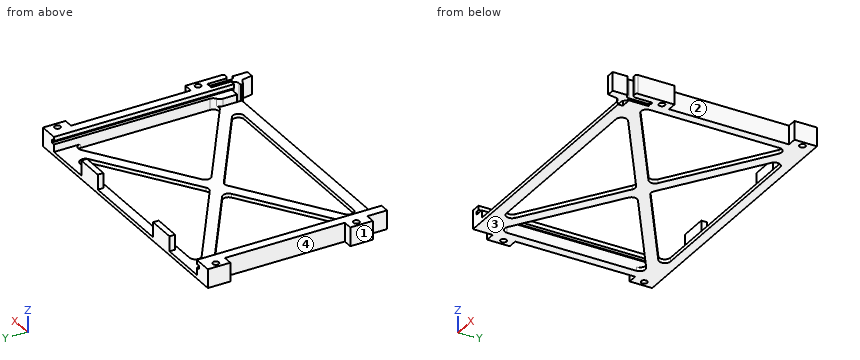
from build123d import *

# Parameters (mm, degrees)
BOSS_EXTRUDE1_DEPTH     = 10
SKETCH3_W               = 134.5
SKETCH3_H               = 1.8
CUT_EXTRUDE1_DEPTH      = 170.435828561
SKETCH5_W               = 140.5
SKETCH5_H               = 6
BOSS_EXTRUDE3_DEPTH     = 2
CUT_EXTRUDE2_DEPTH      = 170.435828561
FILLET1_R               = 3
BOSS_EXTRUDE2_OUTLINE_W = 5
BOSS_EXTRUDE2_OUTLINE_H = 12
BOSS_EXTRUDE2_OUTLINE_R = 1.6
BOSS_EXTRUDE2_DEPTH     = 10
SKETCH7_W               = 130.5
SKETCH7_H               = 5
CUT_EXTRUDE3_DEPTH      = 8
SKETCH8_W               = 15
SKETCH8_H               = 3
BOSS_EXTRUDE4_DEPTH     = 8
BOSS_EXTRUDE5_DEPTH     = 4
FILLET2_R               = 3


# Read off the part's stored shape, not the designer's step: Boss-Extrude2
with BuildPart() as part:
    # Sketch2 → Boss-Extrude1 (new body)
    with BuildSketch(Plane.XY):
        Polygon((2, 0), (-3, 0), (-3, 98.5), (137.5, 98.5), (137.5, 0), (132.5, 0), (132.5, 93.5), (2, 93.5), align=None)
    extrude(amount=BOSS_EXTRUDE1_DEPTH)

    # Sketch3 → Cut-Extrude1 (cut, through all)
    with BuildSketch(Plane.XZ):
        with Locations((67.25, 6.9)):
            Rectangle(SKETCH3_W, SKETCH3_H)
    extrude(amount=-CUT_EXTRUDE1_DEPTH, mode=Mode.SUBTRACT)

    # Sketch5 → Boss-Extrude3 (add)
    with BuildSketch(Plane(origin=(0, 0, 0), x_dir=(-1, 0, 0), z_dir=(0, 0, -1))):
        with Locations((-67.25, 3)):
            Rectangle(SKETCH5_W, SKETCH5_H)
        Polygon((-0.329295866, 8.49173588), (-130.829295866, 95.99173588), (-134.170704134, 91.00826412), (-3.670704134, 3.50826412), align=None)
        Polygon((-3.670704134, 95.99173588), (-134.170704134, 8.49173588), (-130.829295866, 3.50826412), (-0.329295866, 91.00826412), align=None)
    extrude(amount=-BOSS_EXTRUDE3_DEPTH)

    # Sketch4 → Cut-Extrude2 (cut, through all)
    with BuildSketch(Plane.XY):
        with BuildLine():
            ThreePointArc((132, 0), (133.457737974, 0.468990399), (134.368543856, 1.7))
            Line((134.368543856, 1.7), (135, 1.7))
            ThreePointArc((135, 1.7), (135.707106781, 1.992893219), (136, 2.7))
            Line((136, 2.7), (136, 13))
            Line((136, 13), (135.2, 13))
            Line((135.2, 13), (135.2, 2.5))
            Line((135.2, 2.5), (129.5, 2.5))
            Line((129.5, 2.5), (129.5, 0))
            Line((129.5, 0), (130.5, 0))
            Line((130.5, 0), (132, 0))
        make_face()
        with BuildLine():
            ThreePointArc((141.5, 2), (142.207106781, 2.292893219), (142.5, 3))
            Line((142.5, 3), (142.5, -0.5))
            Line((142.5, -0.5), (139.0272352, -0.5))
            Line((139.0272352, -0.5), (138.8, -0.5))
            ThreePointArc((138.8, -0.5), (137.385786438, 0.085786438), (136.8, 1.5))
            Line((136.8, 1.5), (136.8, 12))
            ThreePointArc((136.8, 12), (137.092893219, 12.707106781), (137.8, 13))
            Line((137.8, 13), (138.3, 13))
            ThreePointArc((138.3, 13), (138.653553391, 12.853553391), (138.8, 12.5))
            Line((138.8, 12.5), (138.8, 4))
            ThreePointArc((138.8, 4), (139.385786438, 2.585786438), (140.8, 2))
            Line((140.8, 2), (141.5, 2))
        make_face()
    extrude(amount=CUT_EXTRUDE2_DEPTH, mode=Mode.SUBTRACT)

    # Fillet1
    fillet1_edges = [part.edges().sort_by_distance(p)[0] for p in [
        (132.5, 89.888060199, 1),
        (72.636950218, 49.75, 1),
        (61.863049782, 49.75, 1),
        (67.25, 53.361939801, 1),
        (2, 89.888060199, 1),
        (127.113049782, 93.5, 1),
        (7.386950218, 6, 1),
        (2, 9.611939801, 1),
        (132.5, 9.611939801, 1),
        (67.25, 46.138060199, 1),
        (127.113049782, 6, 1),
        (7.386950218, 93.5, 1),
    ]]
    fillet(fillet1_edges, radius=FILLET1_R)

    # Boss-Extrude2 outline → Boss-Extrude2 (add)
    # profile 1 of 5: a face of its own
    with BuildSketch(Plane.XY):
        with BuildLine():
            Line((134.5, 1.7), (134.368543856, 1.7))
            ThreePointArc((134.368543856, 1.7), (133.457737974, 0.468990399), (132, 0))
            Line((132, 0), (130.5, 0))
            Line((130.5, 0), (130.5, -1.2))
            Line((130.5, -1.2), (134.0272352, -2.83697044))
            Line((134.0272352, -2.83697044), (135.0272352, -8.5))
            Line((135.0272352, -8.5), (139.0272352, -8.5))
            Line((139.0272352, -8.5), (139.0272352, -0.5))
            Line((139.0272352, -0.5), (138.8, -0.5))
            ThreePointArc((138.8, -0.5), (138.092893219, -0.370828693), (137.477124345, 1e-09))
            Line((137.477124345, 1e-09), (134.5, 0))
            Line((134.5, 0), (134.5, 1.7))
        make_face()
    # profile 2 of 5: a face of its own
    with BuildSketch(Plane.XY):
        with Locations((-5.5, 16.5)):
            Rectangle(BOSS_EXTRUDE2_OUTLINE_W, BOSS_EXTRUDE2_OUTLINE_H)
        with Locations((-5, 17.5)):
            Circle(BOSS_EXTRUDE2_OUTLINE_R, mode=Mode.SUBTRACT)
    # profile 3 of 5: a face of its own
    with BuildSketch(Plane.XY):
        with Locations((-5.5, 92.5)):
            Rectangle(BOSS_EXTRUDE2_OUTLINE_W, BOSS_EXTRUDE2_OUTLINE_H)
        with Locations((-5, 92.5)):
            Circle(BOSS_EXTRUDE2_OUTLINE_R, mode=Mode.SUBTRACT)
    # profile 4 of 5: a face of its own
    with BuildSketch(Plane.XY):
        with Locations((140, 92.5)):
            Rectangle(BOSS_EXTRUDE2_OUTLINE_W, BOSS_EXTRUDE2_OUTLINE_H)
        with Locations((139.5, 92.5)):
            Circle(BOSS_EXTRUDE2_OUTLINE_R, mode=Mode.SUBTRACT)
    # profile 5 of 5: a face of its own
    with BuildSketch(Plane.XY):
        with BuildLine():
            Line((137.8, 13), (138.3, 13))
            ThreePointArc((138.3, 13), (138.653553391, 12.853553391), (138.8, 12.5))
            Line((138.8, 12.5), (138.8, 4))
            ThreePointArc((138.8, 4), (139.385786438, 2.585786438), (140.8, 2))
            Line((140.8, 2), (141.5, 2))
            ThreePointArc((141.5, 2), (142.207106781, 2.292893219), (142.5, 3))
            Line((142.5, 3), (142.5, 22.5))
            Line((142.5, 22.5), (137.5, 22.5))
            Line((137.5, 22.5), (137.5, 12.953939201))
            ThreePointArc((137.5, 12.953939201), (137.648242301, 12.988417726), (137.8, 13))
        make_face()
        with Locations((139.5, 17.5)):
            Circle(BOSS_EXTRUDE2_OUTLINE_R, mode=Mode.SUBTRACT)
    extrude(amount=BOSS_EXTRUDE2_DEPTH)

    # Sketch7 → Cut-Extrude3 (cut)
    with BuildSketch(Plane.XY.offset(10)):
        with Locations((67.25, 96)):
            Rectangle(SKETCH7_W, SKETCH7_H)
    extrude(amount=-CUT_EXTRUDE3_DEPTH, mode=Mode.SUBTRACT)

    # Sketch8 → Boss-Extrude4 (add)
    with BuildSketch(Plane.XY.offset(2)):
        with Locations((34.5, 97)):
            Rectangle(SKETCH8_W, SKETCH8_H)
        with Locations((100, 97)):
            Rectangle(SKETCH8_W, SKETCH8_H)
    extrude(amount=BOSS_EXTRUDE4_DEPTH)

    # Sketch9 → Boss-Extrude5 (add)
    with BuildSketch(Plane.XY.offset(2)):
        with BuildLine():
            ThreePointArc((132.5, 15.235373856), (131.621320344, 13.114053512), (129.5, 12.235373856))
            Line((129.5, 12.235373856), (129.5, 2.5))
            Line((129.5, 2.5), (132.5, 2.5))
            Line((132.5, 2.5), (132.5, 15.235373856))
        make_face()
        with BuildLine():
            Line((2, 0), (5, 0))
            Line((5, 0), (5, 12.235373856))
            ThreePointArc((5, 12.235373856), (2.878679656, 13.114053512), (2, 15.235373856))
            Line((2, 15.235373856), (2, 0))
        make_face()
    extrude(amount=BOSS_EXTRUDE5_DEPTH)

    # Fillet2
    fillet2_edges = [part.edges().sort_by_distance(p)[0] for p in [
        (5, 12.235373856, 4),
        (129.5, 12.235373856, 4),
    ]]
    fillet(fillet2_edges, radius=FILLET2_R)


solid = part.part
Verification items for the finished model (mm, model axes). Face numbers are marked on the shaded views. A direction names the side the tool comes from. Give positions to 0.01 mm unless a question says otherwise; leave off trailing zeros. Loops run counter-clockwise (first coordinate to the right, second up) from the corner with the lowest first, then second, coordinate; pieces in that order, holes last.
1) Sectioned sample at A-A, the plane x = -5. Enter the section's corners in (y, z), then the cut area to 3 significant figures.
2) Set-up check for the marked faces 1 and 2: record each of +Z, -Z, +X, -X, +Y, -Y from which the full face is reachable in a straight line by a thin tool's end or side.
3) Sectioned sample at C-C, the plane y = 17.5. Count the separate pieces of the cut face and the enclosed holes in it, then the cut area to 3 significant figures.
4) Thickness scan on line 1 along Y through (x, z) = (-5, 2.25); line 2 along X through (y, z) = (92.5, 3.75); line 3 along X through (y, z) = (10, 9.25). Record the ranges inside material, lowest first.
5) Depth check by flat-ended pin: pin 1 Ø1.6 at (x, y) = (1, 71) entering from -Z; pin 2 Ø1.9 at (x, y) = (139.5, 17.5) entering from -Z; pin 3 Ø2 at (y, z) = (9, 4.5) entering from -X; pin 4 Ø1.5 at (y, z) = (78.5, 2.5) entering from +X. Enter the tip coordinate at first touch or a pass-through.
6) Sectioned sample at B-B, the plane y = 39.5. Enter the section's corners in (x, z).
7) Sectioned sample at D-D, the plane x = 99. Enter the section's corners in (y, z), then the cut area to 3 significant figures.
8) Draft check along Y on the marked faces 3 and 4. Enter one of: pulls with the +Y half, pulls with the -Y half, needs draft (parallel to the pull), parting line crosses it, or undercut.
Answers:
1. outline: (10.5, 0) - (15.9, 0) - (15.9, 10) - (10.5, 10) - close; (19.1, 0) - (22.5, 0) - (22.5, 10) - (19.1, 10) - close; (86.5, 0) - (90.9, 0) - (90.9, 10) - (86.5, 10) - close; (94.1, 0) - (98.5, 0) - (98.5, 10) - (94.1, 10) - close
1. area: 176 mm2
2. face 1: +Z, -Z, -X, +Y, -Y
2. face 2: +Z, -Z, +X
3. separate pieces: 6
3. enclosed holes: 0
3. area: 172 mm2
4. line 1: y = 10.5 to 15.9, 19.1 to 22.5, 86.5 to 90.9, 94.1 to 98.5
4. line 2: x = -8 to -6.6, -3.4 to 2, 132.5 to 137.9, 141.1 to 142.5
4. line 3: x = -3 to 2, 132.5 to 135.2, 136 to 136.8, 138.8 to 142.5
5. pin 1: stops at z = 0
5. pin 2: passes through
5. pin 3: stops at x = -3
5. pin 4: stops at x = 137.5
6. outline: (-3, 0) - (2, 0) - (2, 6) - (0, 6) - (0, 7.8) - (2, 7.8) - (2, 10) - (-3, 10) - close; (46.58, 0) - (57.35, 0) - (57.35, 2) - (46.58, 2) - close; (77.15, 0) - (87.92, 0) - (87.92, 2) - (77.15, 2) - close; (132.5, 0) - (137.5, 0) - (137.5, 10) - (132.5, 10) - (132.5, 7.8) - (134.5, 7.8) - (134.5, 6) - (132.5, 6) - close
7. outline: (0, 0) - (6, 0) - (6, 2) - (0, 2) - close; (24.85, 0) - (32.07, 0) - (32.07, 2) - (24.85, 2) - close; (67.43, 0) - (74.65, 0) - (74.65, 2) - (67.43, 2) - close; (93.5, 0) - (98.5, 0) - (98.5, 10) - (95.5, 10) - (95.5, 2) - (93.5, 2) - close
7. area: 74.9 mm2
8. face 3: needs draft
8. face 4: undercut
